The listing builds one solid part. Answer for the finished solid, in the listing's coordinates (mm). Face numbers are marked on the shaded views. A direction names the side the tool comes from. Round coordinates to 2 decimals unless told otherwise and drop trailing zeros. Write each loop counter-clockwise with the first axis right and the second up, starting at its lowest first coordinate (ties: lowest second). Pieces come first, ordered by that corner, then holes. Notation, with made-up numbers: (88.25, -16) - (143.25, -16) arc R8 ccw to (143.25, -1) - close; hole circle Ø2 at (81.5, -7). An arc over 180 degrees is marked (long way). Use a Markdown table: item, result. Add a question column.
1) Each of these flat-tipped pins is pushed along its axis until it touches: P1, Ø1.5, axis at x = -58, z = -1.5, coming from the -Y side; P2, Ø1.5, axis at y = 0.5, z = -2, coming from the -X side. Where does it stop, or does it pass through?
2) A cutting plane is placed at A-A (z = -3.1). Give the vertices of the cut face in (x, y), then the cut area to 3 significant figures.
3) Find the intervals of material crossed by probe 1 along X at (y, z) = (0.75, -4.2); probe 2 along X at (y, z) = (4.5, -2.8); probe 3 along Y at (x, z) = (-26, -4.1), in increasing order. Write a range as from..to.
4) A cutting plane is placed at B-B (x = -31.5). Give the vertices of the cut face in (y, z), then the cut area to 3 significant figures.
5) A tool of negligible diameter and unlimited length cuts with its end or side. For the marked faces 1, 2 and 3, from which of +Z, -Z, +X, -X, +Y, -Y can it reach the whole face along a straight path? Write none if from no direction.
6) Determine the mould class of the marked faces 4, 5 and 6 for opening direction X: +X half, -X half, draft (parallel to the pull), parting line (faces both ways), or undercut.
Autodesk Inventor part; units mm, degrees
ref_plane "YZ Plane" through (0, 0, 0) normal (1, 0, 0) x (0, 1, 0)
ref_plane "XZ Plane" through (0, 0, 0) normal (0, 1, 0) x (-1, 0, 0)
ref_plane "XY Plane" through (0, 0, 0) normal (0, 0, 1) x (1, 0, 0)
sketch "Эскиз1" plane through (0, 0, 0) normal (0, 1, 0) x (-1, 0, 0)
  line L0 (0, 0) -> (3, 0)
  line L1 (3, 0) -> (3, -5)
  line L2 (3, -5) -> (0, -5)
  line L3 (0, -5) -> (0, 0)
  line L4 (17, 0) -> (20, 0)
  line L5 (20, 0) -> (20, -5)
  line L6 (20, -5) -> (17, -5)
  line L7 (17, -5) -> (17, 0)
  line L8 (34, 0) -> (37, 0)
  line L9 (37, 0) -> (37, -5)
  line L10 (37, -5) -> (34, -5)
  line L11 (34, -5) -> (34, 0)
  line L12 (51, 0) -> (54, 0)
  line L13 (54, 0) -> (54, -5)
  line L14 (54, -5) -> (51, -5)
  line L15 (51, -5) -> (51, 0)
  dimension "d0" = 3
  dimension "d1" = 5
  dimension "d3" = 3
  dimension "d4" = 5
  dimension "d6" = 3
  dimension "d7" = 5
  dimension "d9" = 3
  dimension "d10" = 5
extrude "Выдавливание1" add sketch "Эскиз1" along normal blind 1.4
sketch "Эскиз2" plane through (0, 1.4, 0) normal (0, 1, 0) x (1, 0, 0)
  line L0 (0, 0) -> (-66, 0)
  line L1 (-66, 0) -> (-66, 5)
  line L2 (-66, 5) -> (0, 5)
  line L3 (0, 5) -> (0, 0)
  dimension "d13" = 5
  dimension "d14" = 66
extrude "Выдавливание2" add sketch "Эскиз2" along normal blind 5
fillet "Сопряжение1" radius 2 1 edges at (0, 6.4, -2.5)
properties part number "Bus_copper_bottom" material "Медь"
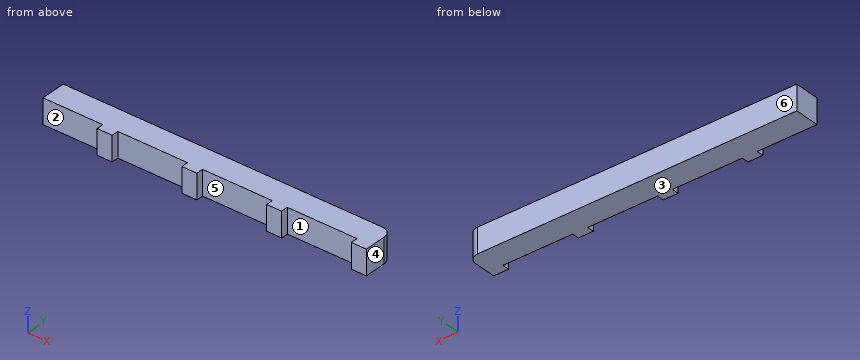
Entries:
| question | item | result |
|---|---|---|
| 1 | P1 | stops at y = 1.4 |
| 1 | P2 | stops at x = -54 |
| 2 | outline | (-66, 1.4) - (-54, 1.4) - (-54, 0) - (-51, 0) - (-51, 1.4) - (-37, 1.4) - (-37, 0) - (-34, 0) - (-34, 1.4) - (-20, 1.4) - (-20, 0) - (-17, 0) - (-17, 1.4) - (-3, 1.4) - (-3, 0) - (0, 0) - (0, 4.4) arc R2 ccw to (-2, 6.4) - (-66, 6.4) - close |
| 2 | area | 346 mm² |
| 3 | probe 1 | x = -54..-51, -37..-34, -20..-17, -3..0 |
| 3 | probe 2 | x = -66..0 |
| 3 | probe 3 | y = 1.4..6.4 |
| 4 | outline | (1.4, -5) - (6.4, -5) - (6.4, 0) - (1.4, 0) - close |
| 4 | area | 25.0 mm² |
| 5 | face 1 | +Z, -Z, -Y |
| 5 | face 2 | +Z, -Z, -X, -Y |
| 5 | face 3 | -Z, +X, -X, +Y, -Y |
| 6 | face 4 | +X half |
| 6 | face 5 | undercut |
| 6 | face 6 | draft |
